Geometry: see drawing. Coordinates: mm, zero at the bounding-box minimum. Coordinates: 2 decimals unless noted, no trailing zeros. Write each loop counter-clockwise with the first axis right and the second up, starting at its lowest first coordinate (ties: lowest second). Pieces come first, ordered by that corner, then holes. Notation, with made-up numbers: (-28.5, 23.25) - (-18.5, 23.25) arc R29 cw to (-18.5, 50.25) - close; hole circle Ø4 at (12, 77). An arc over 180 degrees is marked (long way). Use a Markdown table: item, result. Add a question column.
Q1. Section query B-B (z = 5). Return the cut outline in (x, y), then the cut area to 3 significant figures.
Q2. Section query D-D (x = 19). Return the cut outline in (y, z), then the cut area to 3 significant figures.
Q3. Section query A-A (y = 9). Return the cut outline in (x, z).
Q4. Material intervals for probe 1 along Y at (x, z) = (26, 2); probe 2 along Z at (x, y) = (19, 6.5); probe 3 along X at (y, z) = (9, 4), sorted ascending. Write a range as from..to.
Q5. Section query C-C (x = 26). Return the cut outline in (y, z).
Q6. Mould query, pull axis X, two halves, no side actions, for the marked faces 1, 2, 3 and 4. Classes: released by +X, released by -X, zero draft, split by the parting line, or undercut.
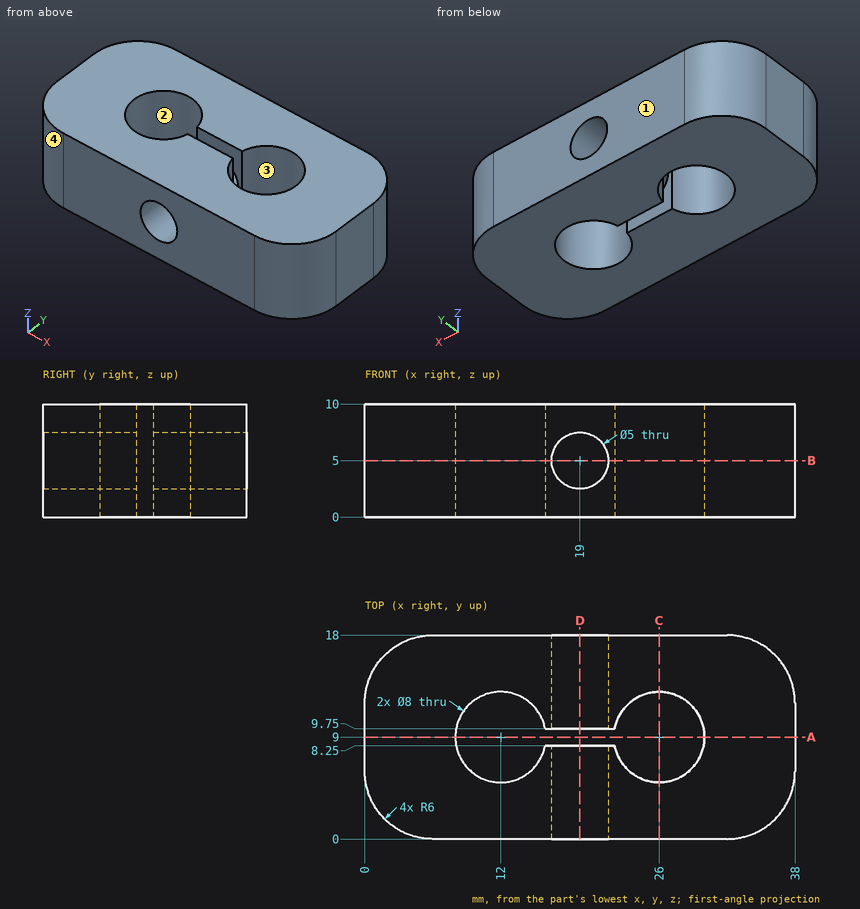
Values follow:
| question | item | result |
|---|---|---|
| 1 | outline | (0, 6) arc R6 ccw to (6, 0) - (16.5, 0) - (16.5, 8.25) - (15.93, 8.25) arc R4 cw (long way) to (15.93, 9.75) - (16.5, 9.75) - (16.5, 18) - (6, 18) arc R6 ccw to (0, 12) - close; (21.5, 0) - (32, 0) arc R6 ccw to (38, 6) - (38, 12) arc R6 ccw to (32, 18) - (21.5, 18) - (21.5, 9.75) - (22.07, 9.75) arc R4 cw (long way) to (22.07, 8.25) - (21.5, 8.25) - close |
| 1 | area | 461 mm2 |
| 2 | outline | (0, 0) - (8.25, 0) - (8.25, 2.5) - (0, 2.5) - close; (0, 7.5) - (8.25, 7.5) - (8.25, 10) - (0, 10) - close; (9.75, 0) - (18, 0) - (18, 2.5) - (9.75, 2.5) - close; (9.75, 7.5) - (18, 7.5) - (18, 10) - (9.75, 10) - close |
| 2 | area | 82.5 mm2 |
| 3 | outline | (0, 0) - (8, 0) - (8, 10) - (0, 10) - close; (30, 0) - (38, 0) - (38, 10) - (30, 10) - close |
| 4 | probe 1 | 0..5, 13..18 |
| 4 | probe 2 | 0..2.5, 7.5..10 |
| 4 | probe 3 | 0..8, 30..38 |
| 5 | outline | (0, 0) - (5, 0) - (5, 10) - (0, 10) - close; (13, 0) - (18, 0) - (18, 10) - (13, 10) - close |
| 6 | face 1 | zero draft |
| 6 | face 2 | undercut |
| 6 | face 3 | undercut |
| 6 | face 4 | released by -X |
